Part print with two shaded views. Sizes in mm from the minimum x, y, z corner. A direction names the side the tool comes from. Give positions to 0.01 mm unless a question says otherwise; leave off trailing zeros. Order: outer loops, then holes, each group sorted by start corner. A loop starts at its lowest first (then second) coordinate and runs counter-clockwise, first axis right, second up. Notation, with made-up numbers: (-32, 45) -> (24, 45) arc R19 cw to (24, 70) -> close; hole circle Ø11 at (-23.75, -15). An arc over 180 degrees is marked (long way). Answer as CSV lines item,"result".
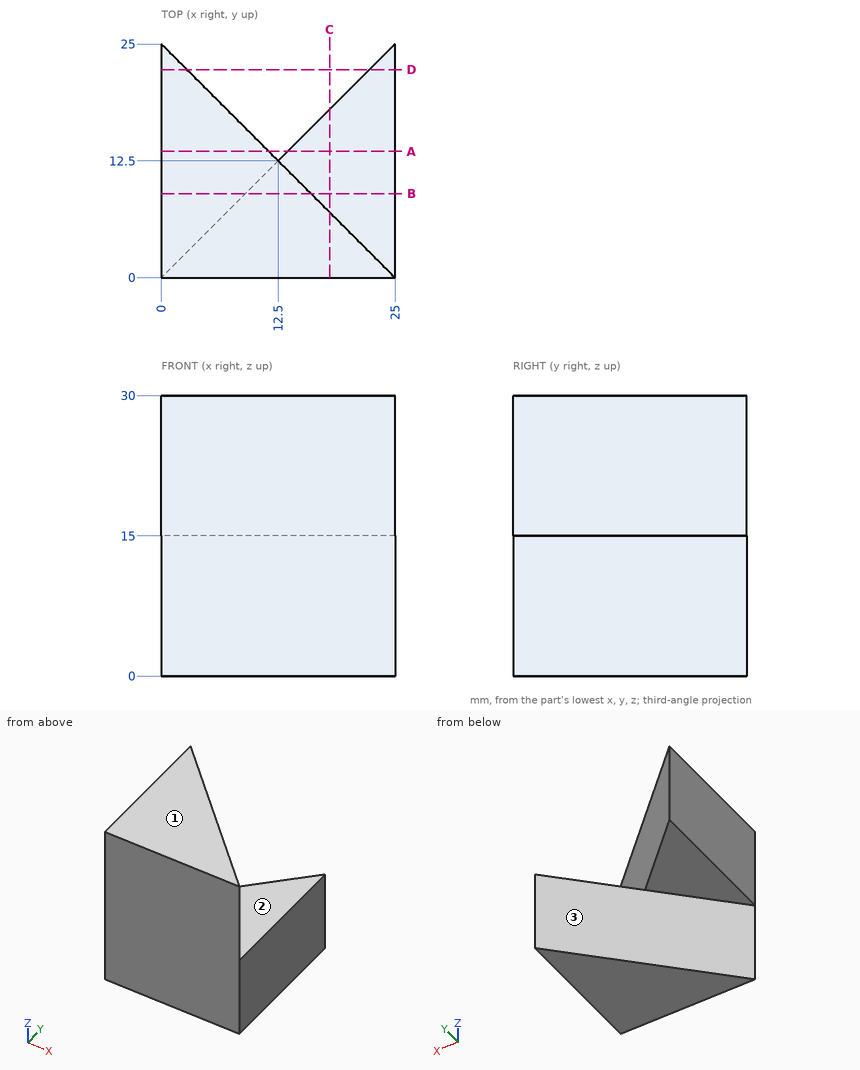
1) Band-saw the part on D-D, the plane y = 22.25. Write the cut outline in (x, z).
Data:
outline,"(0, 15) -> (2.75, 15) -> (2.75, 30) -> (0, 30) -> close; (22.25, 0) -> (25, 0) -> (25, 15) -> (22.25, 15) -> close"
2) Band-saw the part on A-A, the plane y = 13.5. Write the cut outline in (x, z), then the cut area to 3 significant figures.
Data:
outline,"(0, 15) -> (11.5, 15) -> (11.5, 30) -> (0, 30) -> close; (13.5, 0) -> (25, 0) -> (25, 15) -> (13.5, 15) -> close"
area,"345 mm2"
3) Band-saw the part on B-B, the plane y = 9. Write the cut outline in (x, z), then the cut area to 3 significant figures.
Data:
outline,"(0, 15) -> (9, 15) -> (9, 0) -> (25, 0) -> (25, 15) -> (16, 15) -> (16, 30) -> (0, 30) -> close"
area,"480 mm2"
4) Pin check, flat tips, straight feed: P1, Ø3, axis at x = 10, z = 4, coming from the +Y side; P2, Ø8, axis at y = 10, z = 23.5, coming from the +X side; P3, Ø4, axis at x = 18, y = 17.5, coming from the +Z side. Stop position of each tip, or through.
Data:
P1,"stops at y = 11.5"
P2,"stops at x = 19"
P3,"stops at z = 15"
5) Wall check: line 1 along Z through (x, y) = (11.25, 12.75); line 2 along Z through (x, y) = (23.25, 18.25); line 3 along Y through (x, z) = (11, 8.25). Give the ranges that are in metal, low to high. Write a range as [from, to].
Data:
line 1,"z = [15, 30]"
line 2,"z = [0, 15]"
line 3,"y = [0, 11]"
6) Which spindle directions (+Z, -Z, +X, -X, +Y, -Y) get a long thin tool onto all of the face, cutting with end or side? Do the marked faces 1, 2 and 3. Say none if no direction does.
Data:
face 1,"+Z, +X, -X, +Y, -Y"
face 2,"+Z, +X, +Y"
face 3,"-Z, -X, +Y"
7) Band-saw the part on C-C, the plane x = 18. Write the cut outline in (y, z), then the cut area to 3 significant figures.
Data:
outline,"(0, 0) -> (18, 0) -> (18, 15) -> (7, 15) -> (7, 30) -> (0, 30) -> close"
area,"375 mm2"
